Geometry: final body of the model. Coordinates: model frame, mm. A direction names the side the tool comes from. Coordinates: 2 decimals unless noted, no trailing zeros. Write each loop counter-clockwise with the first axis right and the second up, starting at its lowest first coordinate (ties: lowest second). Pieces come first, ordered by that corner, then holes. Notation, with made-up numbers: M 17.25,89.25 L 48.25,89.25 A19 cw 48.25,124.25 Z; hole C 54,20 d2. An arc over 180 degrees is marked long. Write item = value, one per line. Start each with the question number.
Item 1: Section A-A on z = 20. Output: boundary loops of the cut face in (x, y), plus the area to 3 significant figures.
Item 2: Pull-direction query (Y, two-part tool) for faces 4 (the flat face through (-2, 60, 20)), 5 (the flat face through (-59, -1.7, 8)), 6 (the cylindrical face through (76.098, -58.479, 19.199)); classes: +Y half, -Y half, draft (parallel to the pull), parting line (faces both ways), or undercut.
Item 3: Section D-D on z = 31.5. Output: boundary loops of the cut face in (x, y), plus the area to 3 significant figures.
Item 4: Section B-B on x = 70. Output: boundary loops of the cut face in (y, z).
Item 5: Reachability of faces 1 (the cylindrical face through (-56, -3, 5)), 2 (the flat face through (-110, 12, 20)), 3 (the flat face through (-109, -27, 9)) from +Z, -Z, +X, -X, +Y, -Y: full face, straight path, thin tool, end or side. Return the list, or none.
Item 6: Ray query, L1, parallel to X at y = -21, z = 38; L2, parallel to Y at x = 83, z = 37; L3, parallel to X at y = -58.65, z = 20. Return the intervals inside material, ascending. Write a range as [from, to].
Item 7: Section C-C on y = -11. Output: boundary loops of the cut face in (x, z).
Item 8: First-contact query: pin 1 Ø1.3 at (x, y) = (-59, -52) entering from +Z; pin 2 Ø1.8 at (x, y) = (-2, -51.5) entering from +Z. Flat tips, straight axial feed; report the tip coordinate or a pass-through.
from build123d import *

# Parameters (mm, degrees)
SKETCH_1_W          = 220
SKETCH_1_H          = 120
ENCLOSURE_DEPTH     = 40
CAVITY_START        = 3
SKETCH_2_W          = 214
SKETCH_2_H          = 114
CAVITY_DEPTH        = 37
SKETCH_3_R          = 3
STANDOFF_DEPTH      = 8
STANDOFFHOLE_START  = 3
SKETCH_4_R          = 1.1
STANDOFFHOLE_DEPTH  = 5
SKETCH_5_R          = 3
EXTRUDE_3_DEPTH     = 8
CUT_EXTRUDE_START   = 3
SKETCH_6_R          = 1.1
CUT_EXTRUDE_3_DEPTH = 5
SKETCH_7_R          = 3
EXTRUDE_4_DEPTH     = 8
SKETCH_8_R          = 1
CUT_EXTRUDE_4_DEPTH = 5
SKETCH_9_R          = 3
EXTRUDE_5_DEPTH     = 8
SKETCH_10_R         = 1
CUT_EXTRUDE_5_DEPTH = 5
SKETCH_11_R         = 6.15
BUTTONHOLE_DEPTH    = 61
PORT_START          = 9
SKETCH_12_W         = 7
SKETCH_12_H         = 60
PORT_DEPTH          = 16


with BuildPart() as part:
    # 草图1 → Enclosure (new body)
    with BuildSketch(Plane.XY):
        Rectangle(SKETCH_1_W, SKETCH_1_H)
    extrude(amount=ENCLOSURE_DEPTH)

    # 草图2 → Cavity (cut)
    with BuildSketch(Plane.XY.offset(CAVITY_START)):
        Rectangle(SKETCH_2_W, SKETCH_2_H)
    extrude(amount=CAVITY_DEPTH, mode=Mode.SUBTRACT)

    # 草图3 → Standoff (add)
    with BuildSketch(Plane.XY):
        with Locations(Location((-59, -52, 0), (0, 0, 180))):
            Circle(SKETCH_3_R)
    extrude(amount=STANDOFF_DEPTH)

    # 草图4 → StandoffHole (cut)
    with BuildSketch(Plane.XY.offset(STANDOFFHOLE_START)):
        with Locations((-59, -52)):
            Circle(SKETCH_4_R)
    extrude(amount=STANDOFFHOLE_DEPTH, mode=Mode.SUBTRACT)

    # 草图5 → 凸台-拉伸3 (add)
    with BuildSketch(Plane.XY):
        with Locations(Location((-59, -3, 0), (0, 0, 180))):
            Circle(SKETCH_5_R)
    extrude(amount=EXTRUDE_3_DEPTH)

    # 草图6 → 切除-拉伸3 (cut)
    with BuildSketch(Plane.XY.offset(CUT_EXTRUDE_START)):
        with Locations((-59, -3)):
            Circle(SKETCH_6_R)
    extrude(amount=CUT_EXTRUDE_3_DEPTH, mode=Mode.SUBTRACT)

    # 草图7 → 凸台-拉伸4 (add)
    with BuildSketch(Plane.XY):
        with Locations(Location((-1, -52, 0), (0, 0, 180))):
            Circle(SKETCH_7_R)
    extrude(amount=EXTRUDE_4_DEPTH)

    # 草图8 → 切除-拉伸4 (cut)
    with BuildSketch(Plane.XY.offset(CUT_EXTRUDE_START)):
        with Locations((-1, -52)):
            Circle(SKETCH_8_R)
    extrude(amount=CUT_EXTRUDE_4_DEPTH, mode=Mode.SUBTRACT)

    # 草图9 → 凸台-拉伸5 (add)
    with BuildSketch(Plane.XY):
        with Locations(Location((-1, -3, 0), (0, 0, 180))):
            Circle(SKETCH_9_R)
    extrude(amount=EXTRUDE_5_DEPTH)

    # 草图10 → 切除-拉伸5 (cut)
    with BuildSketch(Plane.XY.offset(CUT_EXTRUDE_START)):
        with Locations((-1, -3)):
            Circle(SKETCH_10_R)
    extrude(amount=CUT_EXTRUDE_5_DEPTH, mode=Mode.SUBTRACT)

    # 草图11 → ButtonHole (cut)
    with BuildSketch(Plane(origin=(0, 0, 0), x_dir=(1, 0, 0), z_dir=(0, 1, 0))):
        with Locations(Location((70, -20, 0), (0, 0, 270))):
            Circle(SKETCH_11_R)
    extrude(amount=-BUTTONHOLE_DEPTH, mode=Mode.SUBTRACT)

    # 草图12 → Port (cut)
    with BuildSketch(Plane.XY.offset(PORT_START)):
        with Locations((-108.5, -27.5)):
            Rectangle(SKETCH_12_W, SKETCH_12_H)
    extrude(amount=PORT_DEPTH, mode=Mode.SUBTRACT)


solid = part.part
Responses:
q1.outline = M -110,-60 L 63.85,-60 L 63.85,-57 L -105,-57 L -105,-57.5 L -110,-57.5 Z; M -110,2.5 L -107,2.5 L -107,57 L 107,57 L 107,-57 L 76.15,-57 L 76.15,-60 L 110,-60 L 110,60 L -110,60 Z
q1.area = 1,790 mm²
q2.face_4 = +Y half
q2.face_5 = undercut
q2.face_6 = draft
q3.outline = M -110,-60 L 110,-60 L 110,60 L -110,60 Z; hole M -107,-57 L 107,-57 L 107,57 L -107,57 Z
q3.area = 2,000 mm²
q4.outline = M -60,0 L 60,0 L 60,40 L 57,40 L 57,3 L -57,3 L -57,13.85 L -60,13.85 Z; M -60,26.15 L -57,26.15 L -57,40 L -60,40 Z
q5.face_1 = +Z
q5.face_2 = +Z, -Z, -X, +Y, -Y
q5.face_3 = -X
q6.L1 = [-110, -107], [107, 110]
q6.L2 = [-60, -57], [57, 60]
q6.L3 = [-110, 63.85], [76.15, 110]
q7.outline = M -110,0 L 110,0 L 110,40 L 107,40 L 107,3 L -107,3 L -107,9 L -110,9 Z; M -110,25 L -107,25 L -107,40 L -110,40 Z
q8.pin_1 = 3
q8.pin_2 = 8
